Model file for the job. Use its own axes, mm. Round coordinates to 2 decimals unless told otherwise and drop trailing zeros. Order: outer loops, then holes, each group sorted by start corner. A loop starts at its lowest first (then second) coordinate and runs counter-clockwise, first axis right, second up. Notation, with made-up numbers: (42, -6) -> (64, -6) arc R16 ccw to (64, 16) -> close; hole circle Ø1 at (2.5, 34.5). An arc over 180 degrees is marked (long way). Answer as CSV lines item,"result".
```python
from build123d import *

# Parameters (mm, degrees)
IZIM1_W               = 45
IZIM1_H               = 230
TABAN_FLAN_1_DEPTH    = 10
IZIM6_R               = 3.5
KES_EKSTR_ZYON1_DEPTH = 26
IZIM7_R               = 5.5
KES_EKSTR_ZYON2_DEPTH = 10
RADYUS1_R             = 5


# Sheet-metal steps are written as plain solids
with BuildPart() as part:
    # Çizim1 → Taban-Flanş1 (new body)
    with BuildSketch(Plane.XY):
        Rectangle(IZIM1_W, IZIM1_H)
    extrude(amount=-TABAN_FLAN_1_DEPTH)

    # Çizim6 → Kes-Ekstrüzyon1 (cut)
    with BuildSketch(Plane.XY):
        with Locations((7.5, 7.5)):
            Circle(IZIM6_R)
        with Locations((-7.5, 7.5)):
            Circle(IZIM6_R)
        with Locations((7.5, -7.5)):
            Circle(IZIM6_R)
        with Locations((-7.5, -7.5)):
            Circle(IZIM6_R)
    extrude(amount=-KES_EKSTR_ZYON1_DEPTH, mode=Mode.SUBTRACT)

    # Çizim7 → Kes-Ekstrüzyon2 (cut)
    with BuildSketch(Plane.XY):
        with Locations((0, -100)):
            Circle(IZIM7_R)
        with Locations((0, 100)):
            Circle(IZIM7_R)
    extrude(amount=-KES_EKSTR_ZYON2_DEPTH, mode=Mode.SUBTRACT)

    # Radyus1
    radyus1_edges = [part.edges().sort_by_distance(p)[0] for p in [
        (22.5, -115, -5),
        (-22.5, -115, -5),
        (-22.5, 115, -5),
        (22.5, 115, -5),
    ]]
    fillet(radyus1_edges, radius=RADYUS1_R)


solid = part.part
```
Q1. Wall check: L1, parallel to Y at x = 7.5, z = -4; L2, parallel to Y at x = 0.5, z = -8.75. Give the ranges that are in metal, low to high. Write a range as [from, to].
Checks:
L1,"[-115, -11], [-4, 4], [11, 115]"
L2,"[-115, -105.48], [-94.52, 94.52], [105.48, 115]"
Q2. Saw through at B-B (y = 100). Write the cut outline in (x, z), plus the area to 3 significant figures.
Checks:
outline,"(-22.5, -10) -> (-5.5, -10) -> (-5.5, 0) -> (-22.5, 0) -> close; (5.5, -10) -> (22.5, -10) -> (22.5, 0) -> (5.5, 0) -> close"
area,"340 mm²"
Q3. Saw through at A-A (x = 7.5). Write the cut outline in (y, z).
Checks:
outline,"(-115, -10) -> (-11, -10) -> (-11, 0) -> (-115, 0) -> close; (-4, -10) -> (4, -10) -> (4, 0) -> (-4, 0) -> close; (11, -10) -> (115, -10) -> (115, 0) -> (11, 0) -> close"
Q4. Mould opens along X. For faces 1 (the flat face through (0, 2, -10)), 2 (the cylindrical face through (-10.997, -7.346, -4.93)), 3 (the cylindrical face through (21, 113.57, -5.07)) say: +X half, -X half, draft (parallel to the pull), parting line (faces both ways), or undercut.
Checks:
face 1,"draft"
face 2,"undercut"
face 3,"+X half"
Q5. Saw through at C-C (z = -1.75). Write the cut outline in (x, y), plus the area to 3 significant figures.
Checks:
outline,"(-22.5, -110) arc R5 ccw to (-17.5, -115) -> (17.5, -115) arc R5 ccw to (22.5, -110) -> (22.5, 110) arc R5 ccw to (17.5, 115) -> (-17.5, 115) arc R5 ccw to (-22.5, 110) -> close; hole circle Ø7 at (-7.5, -7.5); hole circle Ø7 at (-7.5, 7.5); hole circle Ø11 at (0, -100); hole circle Ø11 at (0, 100); hole circle Ø7 at (7.5, -7.5); hole circle Ø7 at (7.5, 7.5)"
area,"9,980 mm²"
Q6. Saw through at D-D (y = 7.5). Write the cut outline in (x, z), plus the area to 3 significant figures.
Checks:
outline,"(-22.5, -10) -> (-11, -10) -> (-11, 0) -> (-22.5, 0) -> close; (-4, -10) -> (4, -10) -> (4, 0) -> (-4, 0) -> close; (11, -10) -> (22.5, -10) -> (22.5, 0) -> (11, 0) -> close"
area,"310 mm²"
Q7. Flat gauge pin, fed straight in: pin 1 (9 mm diameter, centred on x = 0, y = 100, fed in from -Z). Where does the tip first touch, or does it go through?
Checks:
pin 1,"through"
